Here's how the part is built. I have some questions about the finished solid (model axes, mm). A direction names the side the tool comes from. Round coordinates to 2 decimals unless told otherwise and drop trailing zeros. Loops run counter-clockwise (first coordinate to the right, second up) from the corner with the lowest first, then second, coordinate; pieces in that order, holes last. Notation, with made-up numbers: M 18.5,-26.75 L 70.5,-26.75 A19 cw 70.5,6.25 Z; hole C 52.25,30.5 d1. An arc over 180 degrees is marked long. Answer as a JSON object with one key per item and string values.
from build123d import *

# Parameters (mm, degrees)
BOSS_EXTRUDE1_DEPTH      = 7
SKETCH1_3_R              = 1.6
BOSS_EXTRUDE2_DEPTH      = 1.5
SKETCH2_W                = 30
SKETCH2_H                = 8.5
BOSS_EXTRUDE3_DEPTH      = 6
BOSS_EXTRUDE4_DEPTH      = 10
BOSS_EXTRUDE4_DEPTH_BACK = 6
SKETCH3_W                = 10
SKETCH3_H                = 6.2


with BuildPart() as part:
    # Sketch1 → Boss-Extrude1 (new body)
    with BuildSketch(Plane.XY):
        Polygon((0, 0), (15, 0), (15, 13), (0, 13), (0, 10), (0, 3), align=None)
    boss_extrude1 = extrude(amount=BOSS_EXTRUDE1_DEPTH)

    # Sketch1<3> → Boss-Extrude2 (add)
    with BuildSketch(Plane.XY):
        with BuildLine():
            Line((0, 10), (-4.041019256, 10))
            ThreePointArc((-4.041019256, 10), (-7.541019256, 6.5), (-4.041019256, 3))
            Line((-4.041019256, 3), (0, 3))
            Line((0, 3), (0, 10))
        make_face()
        with Locations((-4.041019256, 6.5)):
            Circle(SKETCH1_3_R, mode=Mode.SUBTRACT)
    boss_extrude2 = extrude(amount=BOSS_EXTRUDE2_DEPTH)

    # Mirror1: Boss-Extrude1, Boss-Extrude2 across plane
    add(boss_extrude1.mirror(Plane(origin=(15, -13.88108581, 7), x_dir=(0, 0, 1), z_dir=(-1, 0, 0))))
    add(boss_extrude2.mirror(Plane(origin=(15, -13.88108581, 7), x_dir=(0, 0, 1), z_dir=(-1, 0, 0))))

    # Sketch2 → Boss-Extrude3 (add)
    with BuildSketch(Plane.XY.offset(7)):
        with Locations((15, 6.5)):
            Rectangle(SKETCH2_W, SKETCH2_H)
    extrude(amount=BOSS_EXTRUDE3_DEPTH)

    # Sketch3 → Boss-Extrude4 (add, two sides: drawn at the far end of the back side and taken through both)
    with BuildSketch(Plane.XZ.offset(-BOSS_EXTRUDE4_DEPTH_BACK)):
        with Locations((14.510328708, 5.6)):
            Rectangle(SKETCH3_W, SKETCH3_H)
    extrude(amount=BOSS_EXTRUDE4_DEPTH + BOSS_EXTRUDE4_DEPTH_BACK)


solid = part.part
Item 1: I want a section at D-D on y = -4. List the corners of the cut face in (x, z) for me.
Solution:
{"outline": "M 9.51,2.5 L 19.51,2.5 L 19.51,8.7 L 9.51,8.7 Z"}
Item 2: For P1, Ø5, axis at y = -4, z = 4.5, coming from the -X side; P2, Ø3.5, axis at x = -5, y = 8, coming from the +Z side; P3, Ø1.2, axis at x = 31.5, z = 0.5, coming from the -Y side, each with a flat end and sliding along its axis, tell me the tip position at first contact or that it passes through.
Solution:
{"P1": "stops at x = 9.51", "P2": "stops at z = 1.5", "P3": "stops at y = 3"}
Item 3: If I drill on L1, parallel to X at y = 5.75, z = 11; L2, parallel to Z at x = 19, y = -8; L3, parallel to Y at x = 27.5, z = 1.5, over which ranges is the centre line in solid material (lowest first)? Write a range as from..to.
Solution:
{"L1": "x = 0..30", "L2": "z = 2.5..8.7", "L3": "y = 0..13"}
Item 4: I want a section at B-B on x = 25. List the corners of the cut face in (y, z) for me.
Solution:
{"outline": "M 0,0 L 13,0 L 13,7 L 10.75,7 L 10.75,13 L 2.25,13 L 2.25,7 L 0,7 Z"}
Item 5: We'd pull the mould along X, two halves only. Please class faces 1 (the face through (-2, 10, 1)), 2 (the face through (37.54, 6.58, 0.74)), 3 (the face through (-4.39, 4.94, 0.74)): +X half, -X half, draft (parallel to the pull), parting line (faces both ways), or undercut.
Solution:
{"face 1": "draft", "face 2": "+X half", "face 3": "undercut"}
Item 6: I want a section at A-A on y = 6.5. List the corners of the cut face in (x, z) for me.
Solution:
{"outline": "M -7.54,0 L -5.64,0 L -5.64,1.5 L -7.54,1.5 Z; M -2.44,0 L 32.44,0 L 32.44,1.5 L 30,1.5 L 30,13 L 0,13 L 0,1.5 L -2.44,1.5 Z; M 35.64,0 L 37.54,0 L 37.54,1.5 L 35.64,1.5 Z"}
Item 7: I want a section at C-C on z = 5.25. List the corners of the cut face in (x, y) for me, plus the area to 3 significant figures.
Solution:
{"outline": "M 0,0 L 9.51,0 L 9.51,-10 L 19.51,-10 L 19.51,0 L 30,0 L 30,13 L 0,13 Z", "area": "490 mm2"}
Item 8: For faces 4 (the face through (15, 10.75, 10)), 5 (the face through (32, 10, 1)), 6 (the face through (14, -5, 2.5)), 7 (the face through (32, 7, 1.5)), which set-ups out of +Z, -Z, +X, -X, +Y, -Y let a thin tool reach every point of the face, with its end or its side?
Solution:
{"face 4": "+Z, +X, -X, +Y", "face 5": "+Z, -Z, +X, +Y", "face 6": "-Z, +X, -X, -Y", "face 7": "+Z, +X, +Y, -Y"}
